Can you work these out from the model? Positions are in its coordinate system, mm. A direction names the side the tool comes from. Give positions to 0.01 mm unless a question says otherwise; leave off trailing zeros. Write each question's results on one line, items separated by ' | '.
Autodesk Inventor part; units mm, degrees
ref_plane "YZ Plane" through (0, 0, 0) normal (1, 0, 0) x (0, 1, 0)
ref_plane "XZ Plane" through (0, 0, 0) normal (0, 1, 0) x (-1, 0, 0)
ref_plane "XY Plane" through (0, 0, 0) normal (0, 0, 1) x (1, 0, 0)
ref_plane "Work Plane1" through (0, 0, 0) normal (0, 0, 1) x (1, 0, 0)
sketch "Sketch1" plane through (0, 0, 0) normal (0, 0, 1) x (1, 0, 0)
  line L0 (-28, 30) -> (-30, 28)
  line L1 (-30, 28) -> (-30, -28)
  line L2 (-30, -28) -> (-28, -30)
  line L3 (-28, -30) -> (28, -30)
  line L4 (28, -30) -> (30, -28)
  line L5 (30, -28) -> (30, -17.7934)
  line L6 (30, 28) -> (28, 30)
  line L7 (28, 30) -> (17.7934, 30)
  line L8 (-25, -25) -> (25, -25) construction
  line L9 (25, -25) -> (25, 25) construction
  line L10 (25, 25) -> (-25, 25) construction
  line L11 (-25, 25) -> (-25, -25) construction
  line L12 (-25, -25) -> (25, 25) construction
  line L13 (25, -25) -> (-25, 25) construction
  line L14 (30, -17.7934) -> (44, -17.7934)
  line L15 (44, -9.0511) -> (44, -17.7934)
  line L16 (30, -9.0511) -> (44, -9.0511) construction
  line L17 (30, -9.0511) -> (30, 8.3051)
  line L18 (30, 8.3051) -> (44, 8.3051)
  line L19 (44, 19.2331) -> (44, 8.3051)
  line L20 (30, 19.2331) -> (44, 19.2331) construction
  line L21 (30, 28) -> (30, -28)
  line L22 (17.7934, 30) -> (17.7934, 44)
  line L23 (9.0511, 44) -> (17.7934, 44)
  line L24 (9.0511, 30) -> (9.0511, 44) construction
  line L25 (-8.3051, 30) -> (-8.3051, 44)
  line L26 (-19.2331, 44) -> (-8.3051, 44)
  line L27 (-19.2331, 30) -> (-19.2331, 44) construction
  line L28 (-19.2331, 30) -> (-28, 30)
  line L29 (-28, 30) -> (28, 30)
  line L30 (25, 0) -> (-25, 0)
  line L31 (30, 19.2331) -> (30, 28)
  line L32 (9.0511, 30) -> (-8.3051, 30)
  point P0 (0, 0)
  dimension "d0" = 50
  dimension "d1" = 50
extrude "Extrusion1" add sketch "Sketch1" along normal blind 12
sketch "Sketch2" plane through (0, 0, 12) normal (0, 0, 1) x (1, 0, 0)
  line L0 (-25, -25) -> (25, -25)
  line L1 (25, -25) -> (25, 25)
  line L2 (25, 25) -> (-25, 25)
  line L3 (-25, 25) -> (-25, -25)
  line L4 (-25, -25) -> (25, 25) construction
  line L5 (25, -25) -> (-25, 25) construction
  point P0 (0, 0)
  point P1 (25, 0)
  point P2 (-25, 0)
  point P3 (0, 25)
  point P4 (0, -25)
  dimension "d4" = 50
  dimension "d5" = 50
hole "Hole1" at (25, 25, 12) at (25, -25, 12) at (-25, -25, 12) at (-25, 25, 12) at (-25, 0, 12) at (25, 0, 12) at (0, 25, 12) at (0, -25, 12) direction (0, 0, -1) diameter 3.9 depth 10 tip angle 118
properties part number "00_XY_stage-CHUO_SEIKI_LD-647-R1-Bottom"
(1) I need wall thicknesses on L1, parallel to X at y = -25, z = 5.25; L2, parallel to Y at x = 0, z = 6.5. Which ranges of each line are inside material? Lowest first, please. Write a range as from..to.
Data:
L1: x = -30..-26.95, -23.05..-1.95, 1.95..23.05, 26.95..30 | L2: y = -30..-26.95, -23.05..23.05, 26.95..30
(2) Imagine slicing it at A-A, the plane z = 5.25. Count the separate pieces of the cut face and the enclosed holes in it, plus the area to 3 significant figures.
Data:
separate pieces: 1 | enclosed holes: 8 | area: 3,500 mm2
(3) Will these pins go through, and if not, where does the flat tip stop? P1, Ø6, axis at x = 22, y = 9, coming from the -Z side; P2, Ø3.5, axis at x = -25, y = 0, coming from the +Z side.
Data:
P1: stops at z = 0 | P2: stops at z = 1.88
(4) We'd pull the mould along Y, two halves only. Please class faces 3 (the face through (30, 0, 6)), 4 (the face through (23.067, 25.254, 6.93)), 5 (the face through (-29, 29, 6)): +Y half, -Y half, draft (parallel to the pull), parting line (faces both ways), or undercut.
Data:
face 3: draft | face 4: undercut | face 5: +Y half
(5) For faces 1 (the face through (-30, 0, 6)), 2 (the face through (-26.933, 0.254, 6.93)), which set-ups out of +Z, -Z, +X, -X, +Y, -Y let a thin tool reach every point of the face, with its end or its side?
Data:
face 1: +Z, -Z, -X, +Y, -Y | face 2: +Z
